from build123d import *

# Parameters (mm, degrees)
SKETCH2_W           = 40
SKETCH2_H           = 18
SKETCH2_R           = 1.6
BOSS_EXTRUDE1_DEPTH = 5
FILLET1_R           = 3


with BuildPart() as part:
    # Sketch2 → Boss-Extrude1 (new body)
    with BuildSketch(Plane(origin=(0, 0, 0), x_dir=(1, 0, 0), z_dir=(0, 1, 0))):
        with Locations((20, 9)):
            Rectangle(SKETCH2_W, SKETCH2_H)
        with Locations(Location((5.9, 14, 0), (0, 0, 270))):
            Circle(SKETCH2_R, mode=Mode.SUBTRACT)
        with Locations(Location((34.1, 14, 0), (0, 0, 270))):
            Circle(SKETCH2_R, mode=Mode.SUBTRACT)
        with Locations(Location((13.5, 4, 0), (0, 0, 270))):
            Circle(SKETCH2_R, mode=Mode.SUBTRACT)
        with Locations(Location((26.5, 4, 0), (0, 0, 270))):
            Circle(SKETCH2_R, mode=Mode.SUBTRACT)
    extrude(amount=BOSS_EXTRUDE1_DEPTH)

    # Fillet1
    fillet1_edges = [part.edges().sort_by_distance(p)[0] for p in [
        (0, 2.5, -18),
        (40, 2.5, -18),
        (40, 2.5, 0),
        (0, 2.5, 0),
    ]]
    fillet(fillet1_edges, radius=FILLET1_R)


solid = part.part
Source: CAD feature listing. Evaluate the final solid. Frame: model axes, mm. Round coordinates to 2 decimals unless told otherwise and drop trailing zeros. Loops run counter-clockwise (first coordinate to the right, second up) from the corner with the lowest first, then second, coordinate; pieces in that order, holes last. Notation, with made-up numbers: (-38.75, -4.75) - (4.25, -4.75) arc R16 ccw to (4.25, -0.75) - close; hole circle Ø4 at (1, -20.75). An arc over 180 degrees is marked (long way). Write item = value, one per line. Start each with the question number.
Item 1: Section query B-B on x = 34.1. Output: boundary loops of the cut face in (y, z), plus the area to 3 significant figures.
Item 2: Section query D-D on x = 5. Output: boundary loops of the cut face in (y, z), plus the area to 3 significant figures.
Item 3: Section query A-A on y = 1.75. Output: boundary loops of the cut face in (x, z), plus the area to 3 significant figures.
Item 4: Material intervals for line 1 (X direction, y = 2.1, z = -4); line 2 (X direction, y = 1.65, z = -14); line 3 (Z direction, x = 35.5, y = 4.05), sorted ascending.
Item 5: Section query C-C on z = -14. Output: boundary loops of the cut face in (x, y), plus the area to 3 significant figures.
Item 6: Mould query, pull axis X, two halves, no side actions, for faces 1 (the face through (20, 2, -18)), 2 (the face through (5.97, 2.46, -15.6)), 3 (the face through (39.1, 2.54, -0.86)). Classes: released by +X, released by -X, zero draft, split by the parting line, or undercut.
Results list:
q1.outline = (0, -18) - (5, -18) - (5, -15.6) - (0, -15.6) - close; (0, -12.4) - (5, -12.4) - (5, 0) - (0, 0) - close
q1.area = 74.0 mm²
q2.outline = (0, -18) - (5, -18) - (5, -15.32) - (0, -15.32) - close; (0, -12.68) - (5, -12.68) - (5, 0) - (0, 0) - close
q2.area = 76.8 mm²
q3.outline = (0, -15) arc R3 ccw to (3, -18) - (37, -18) arc R3 ccw to (40, -15) - (40, -3) arc R3 ccw to (37, 0) - (3, 0) arc R3 ccw to (0, -3) - close; hole circle Ø3.2 at (5.9, -14); hole circle Ø3.2 at (13.5, -4); hole circle Ø3.2 at (26.5, -4); hole circle Ø3.2 at (34.1, -14)
q3.area = 680 mm²
q4.line_1 = 0 to 11.9, 15.1 to 24.9, 28.1 to 40
q4.line_2 = 0 to 4.3, 7.5 to 32.5, 35.7 to 40
q4.line_3 = -18 to -14.77, -13.23 to 0
q5.outline = (0, 0) - (4.3, 0) - (4.3, 5) - (0, 5) - close; (7.5, 0) - (32.5, 0) - (32.5, 5) - (7.5, 5) - close; (35.7, 0) - (40, 0) - (40, 5) - (35.7, 5) - close
q5.area = 168 mm²
q6.face_1 = zero draft
q6.face_2 = undercut
q6.face_3 = released by +X
